Autodesk Inventor part; units mm, degrees
ref_plane "YZ Plane" through (0, 0, 0) normal (1, 0, 0) x (0, 1, 0)
ref_plane "XZ Plane" through (0, 0, 0) normal (0, 1, 0) x (-1, 0, 0)
ref_plane "XY Plane" through (0, 0, 0) normal (0, 0, 1) x (1, 0, 0)
sketch "Sketch1" plane through (0, 0, 0) normal (0, 1, 0) x (-1, 0, 0)
  line L0 (-1.4187, 3.9318) -> (11.2813, 3.9318)
  line L1 (11.2813, 3.9318) -> (11.2813, -8.7682)
  line L2 (11.2813, -8.7682) -> (-1.4187, -8.7682)
  line L3 (-1.4187, -8.7682) -> (-1.4187, 3.9318)
  point P0 (0, 0)
  dimension "d0" = 12.7
  dimension "d1" = 12.7
extrude "Extrusion1" add sketch "Sketch1" along normal blind 2.54
sketch "Sketch2" plane through (0, 2.54, 0) normal (0, 1, 0) x (1, 0, 0)
  line L0 (-1.1213, -0.7568) -> (-7.4713, -0.7568)
  line L1 (-7.4713, -0.7568) -> (-7.4713, 5.5932)
  line L2 (-7.4713, 5.5932) -> (-1.1213, 5.5932)
  line L3 (-1.1213, 5.5932) -> (-1.1213, -0.7568)
  line L4 (1.4187, 8.7682) -> (-11.2813, 8.7682)
  line L5 (1.4187, -3.9318) -> (1.4187, 8.7682)
  point P0 (0, 0)
  dimension "d4" = 6.35
  dimension "d5" = 6.35
  dimension "d6" = 3.175
  dimension "d7" = 2.54
extrude "Extrusion2" add sketch "Sketch2" along normal blind 16.51
sketch "Sketch3" plane through (-1.1213, 2.54, 0.7568) normal (1, 0, 0) x (0, 0, -1)
  line L0 (0, 16.51) -> (6.35, 16.51)
  line L1 (3.175, 16.51) -> (3.175, 20.32)
  line L2 (3.175, 20.32) -> (5.6637, 20.32)
  point P0 (0.7568, -2.54)
  dimension "d10" = 3.81
ref_plane "Work Plane1" through (-1.1213, 22.86, -4.9069) normal (0.5144958, -0.8574929, 0) x (0, 0, 1)
sketch "Sketch4" plane through (-1.1213, 22.86, -4.9069) normal (0.5144958, -0.8574929, 0) x (0, 0, 1)
  line L0 (-2.5913, 9.9453) -> (7.5687, 9.9453)
  line L1 (7.5687, 9.9453) -> (7.5687, -0.2147)
  line L2 (7.5687, -0.2147) -> (-2.5913, -0.2147)
  line L3 (-2.5913, -0.2147) -> (-2.5913, 9.9453)
  line L4 (5.6637, 7.4053) -> (5.6637, 1.9602)
  line L5 (-0.6863, 7.4053) -> (5.6637, 7.4053)
  point P0 (4.9069, 10.7999)
  dimension "d11" = 10.16
  dimension "d12" = 10.16
  dimension "d13" = 1.905
  dimension "d14" = 2.54
extrude "Extrusion3" add sketch "Sketch4" along normal blind 2.54
sketch "Sketch5" plane through (0, 19.05, 0) normal (0, 1, 0) x (1, 0, 0)
  line L0 (-8.3425, -2.6618) -> (-8.3425, 7.4982)
  line L1 (-8.3425, 7.4982) -> (0.3696, 7.4982)
  line L2 (0.3696, 7.4982) -> (0.3696, -2.6618)
  line L3 (0.3696, -2.6618) -> (-8.3425, -2.6618)
  line L4 (-7.4713, -0.7568) -> (-7.4713, 5.5932)
  line L5 (-2.5344, -0.7568) -> (-7.4713, -0.7568)
  line L6 (-2.5344, 5.5932) -> (-2.5344, -0.7568)
  line L7 (-7.4713, 5.5932) -> (-2.5344, 5.5932)
  line L8 (-1.1213, -0.7568) -> (-2.5344, -0.7568)
  line L9 (-2.5344, -0.7568) -> (-2.5344, 5.5932)
  line L10 (-2.5344, 5.5932) -> (-1.1213, 5.5932)
  line L11 (-1.1213, 5.5932) -> (-1.1213, -0.7568)
  point P0 (0, 0)
extrude "Extrusion4" add sketch "Sketch5" along normal up to next contours L6 L10 L11 L8
properties part number "Plaque"
Source: CAD feature listing. Evaluate the final solid. Frame: model axes, mm. A direction names the side the tool comes from. Round coordinates to 2 decimals unless told otherwise and drop trailing zeros. Loops run counter-clockwise (first coordinate to the right, second up) from the corner with the lowest first, then second, coordinate; pieces in that order, holes last. Notation, with made-up numbers: (66, -30.5) -> (100, -30.5) arc R14 ccw to (100, -8.5) -> close; hole circle Ø6 at (52, 72.25). An arc over 180 degrees is marked (long way). Answer as a JSON object with one key per item and string values. Group by question number.
Q1. Section query A-A (z = 2.25). Output: boundary loops of the cut face in (x, y).
Q2. Ray query, line 1 (Z direction, x = -3.25, y = 11); line 2 (X direction, y = 11.75, z = -3); line 3 (Y direction, x = -4.25, z = -6). Return the intervals inside material, ascending. Write a range as from..to.
Q3. Contact query for flat-ended pins moving along their axis: P1, Ø3, axis at y = 17, z = -1.5, coming from the -X side; P2, Ø3.5, axis at x = -2.5, y = 19.5, coming from the -Z side; P3, Ø6, axis at x = -9, y = 18.5, coming from the +Z side; P4, Ø1, axis at x = -8, y = 20.5, coming from the -Z side. Output: stop coordinate, or through.
Q4. Section query C-C (z = -0.25). Output: boundary loops of the cut face in (x, y), plus the area to 3 significant figures.
Q5. Section query B-B (x = -0.25). Output: boundary loops of the cut face in (y, z).
Q6. Mould query, pull axis Y, two halves, no side actions, for faces 6 (the flat face through (-11.281, 1, -2)), 7 (the flat face through (-4, 11, -5.593)), 8 (the flat face through (-0.293, 21.897, -2.347)). Classes: pulls with the +Y half, pulls with the -Y half, needs draft (parallel to the pull), parting line crosses it, or undercut.
Q7. Access query for faces 1 (the flat face through (-1.121, 11, -2)), 2 (the flat face through (-8, 2.54, -2)), 3 (the flat face through (-4, 11, 0.757)), 4 (the flat face through (-5, 19, 2.662)), 5 (the flat face through (-9.005, 16.669, -2.489)). Directions: +Z, -Z, +X, -X, +Y, -Y. A direction counts if a zero-diameter tool reaches every point of the face in a straight line with its end or side. Return the directions, or none.
Q8. Section query D-D (x = -3.75). Output: boundary loops of the cut face in (y, z).
Completed:
{
 "1": {"outline": "(-11.28, 0) -> (1.42, 0) -> (1.42, 2.54) -> (-11.28, 2.54) -> close; (-9.65, 17.74) -> (-8.34, 15.57) -> (0.37, 20.79) -> (-0.94, 22.97) -> close"},
 "2": {"line 1": "-5.59..0.76", "line 2": "-7.47..-1.12", "line 3": "0..2.54, 18.02..20.98"},
 "3": {"P1": "x = -9.65", "P2": "z = -7.5", "P3": "z = 2.66", "P4": "through"},
 "4": {"outline": "(-11.28, 0) -> (1.42, 0) -> (1.42, 2.54) -> (-1.12, 2.54) -> (-1.12, 19.9) -> (0.37, 20.79) -> (-0.94, 22.97) -> (-9.65, 17.74) -> (-8.34, 15.57) -> (-7.47, 16.09) -> (-7.47, 2.54) -> (-11.28, 2.54) -> close", "area": "156 mm²"},
 "5": {"outline": "(0, -8.77) -> (2.54, -8.77) -> (2.54, 3.93) -> (0, 3.93) -> close; (20.42, -7.5) -> (21.83, -7.5) -> (21.83, 2.66) -> (20.42, 2.66) -> close"},
 "6": {"face 6": "needs draft", "face 7": "undercut", "face 8": "pulls with the +Y half"},
 "7": {"face 1": "+Z, -Z, +X", "face 2": "none", "face 3": "+Z, +X", "face 4": "+Z, +X, -X, +Y", "face 5": "+Z, -Z, -X"},
 "8": {"outline": "(0, -8.77) -> (2.54, -8.77) -> (2.54, -5.59) -> (18.32, -5.59) -> (18.32, -7.5) -> (21.28, -7.5) -> (21.28, 2.66) -> (18.32, 2.66) -> (18.32, 0.76) -> (2.54, 0.76) -> (2.54, 3.93) -> (0, 3.93) -> close"}
}
